Part model, mm, in its own coordinate system. A direction names the side the tool comes from. Round coordinates to 2 decimals unless told otherwise and drop trailing zeros. Loops run counter-clockwise (first coordinate to the right, second up) from the corner with the lowest first, then second, coordinate; pieces in that order, holes last. Notation, with made-up numbers: M 16,-29.5 L 26,-29.5 A16 cw 26,-5.5 Z; hole C -23,-37.75 d7. An arc over 180 degrees is marked long. Write each question's results on one line, items separated by ' | '.
from build123d import *

# Parameters (mm, degrees)
SKETCH1_R           = 1.249999999
BOSS_EXTRUDE1_DEPTH = 6.35


with BuildPart() as part:
    # Sketch1 → Boss-Extrude1 (new body)
    with BuildSketch(Plane.XY):
        with BuildLine():
            Line((200.750613804, 258.978854223), (200.750613804, 219.828854223))
            ThreePointArc((200.750613804, 219.828854223), (201.680549774, 217.583790192), (203.925613804, 216.653854223))
            Line((203.925613804, 216.653854223), (221.575613802, 216.653854223))
            ThreePointArc((221.575613802, 216.653854223), (223.820677833, 217.583790192), (224.750613802, 219.828854223))
            Line((224.750613802, 219.828854223), (224.750613802, 258.978854223))
            ThreePointArc((224.750613802, 258.978854223), (223.820677833, 261.223918253), (221.575613802, 262.153854223))
            Line((221.575613802, 262.153854223), (203.925613804, 262.153854223))
            ThreePointArc((203.925613804, 262.153854223), (201.680549774, 261.223918253), (200.750613804, 258.978854223))
        make_face()
        with Locations((211.950613802, 247.891354224)):
            Circle(SKETCH1_R, mode=Mode.SUBTRACT)
        with Locations((211.950613802, 257.416354224)):
            Circle(SKETCH1_R, mode=Mode.SUBTRACT)
        with BuildLine():
            Line((203.700613802, 221.203854223), (203.700613802, 224.103854225))
            ThreePointArc((203.700613802, 224.103854225), (206.250613802, 226.653854225), (208.800613803, 224.103854225))
            Line((208.800613803, 224.103854225), (208.800613803, 221.203854223))
            ThreePointArc((208.800613803, 221.203854223), (206.250613802, 218.653854223), (203.700613802, 221.203854223))
        make_face(mode=Mode.SUBTRACT)
        with BuildLine():
            Line((216.700613804, 224.103854225), (216.700613804, 221.203854223))
            ThreePointArc((216.700613804, 221.203854223), (219.250613803, 218.653854224), (221.800613802, 221.203854223))
            Line((221.800613802, 221.203854223), (221.800613802, 224.103854225))
            ThreePointArc((221.800613802, 224.103854225), (219.250613803, 226.653854224), (216.700613804, 224.103854225))
        make_face(mode=Mode.SUBTRACT)
    extrude(amount=BOSS_EXTRUDE1_DEPTH)


solid = part.part
Item 1: Band-saw the part on C-C on z = 3. Give the cut face in (x, y) (3 decimals), and give its area (3 significant figures).
Filled sheet:
outline: M 200.751,219.829 A3.175 ccw 203.926,216.654 L 221.576,216.654 A3.175 ccw 224.751,219.829 L 224.751,258.979 A3.175 ccw 221.576,262.154 L 203.926,262.154 A3.175 ccw 200.751,258.979 Z; hole M 203.701,221.204 A2.55 ccw 208.801,221.204 L 208.801,224.104 A2.55 ccw 203.701,224.104 Z; hole C 211.951,247.891 d2.5; hole C 211.951,257.416 d2.5; hole M 216.701,221.204 A2.55 ccw 221.801,221.204 L 221.801,224.104 A2.55 ccw 216.701,224.104 Z | area: 1,000 mm^2
Item 2: Wall check: L1, parallel to Y at x = 212, z = 6.25; L2, parallel to X at y = 223, z = 4.75; L3, parallel to X at y = 226, z = 4. Give the ranges that are in metal, low to high.
Filled sheet:
L1: 216.65 to 246.64, 249.14 to 256.17, 258.67 to 262.15 | L2: 200.75 to 203.7, 208.8 to 216.7, 221.8 to 224.75 | L3: 200.75 to 204.55, 207.96 to 217.55, 220.96 to 224.75
Item 3: Band-saw the part on A-A on y = 223.5. Give the cut face in (x, z).
Filled sheet:
outline: M 200.75,0 L 203.7,0 L 203.7,6.35 L 200.75,6.35 Z; M 208.8,0 L 216.7,0 L 216.7,6.35 L 208.8,6.35 Z; M 221.8,0 L 224.75,0 L 224.75,6.35 L 221.8,6.35 Z
Item 4: Two-plate mould, pull along Y, no slides. Class faces 3 (the cylindrical face through (219.195, 218.654, 3.131)), 4 (the cylindrical face through (201.656, 217.609, 3.131)), 5 (the flat face through (208.801, 223, 3)), 6 (the flat face through (224.751, 239, 3)): +Y half, -Y half, draft (parallel to the pull), parting line (faces both ways), or undercut.
Filled sheet:
face 3: undercut | face 4: -Y half | face 5: undercut | face 6: draft
Item 5: Band-saw the part on B-B on x = 205.5. Give the cut face in (y, z), and give its area (3 significant figures).
Filled sheet:
outline: M 216.65,0 L 218.77,0 L 218.77,6.35 L 216.65,6.35 Z; M 226.54,0 L 262.15,0 L 262.15,6.35 L 226.54,6.35 Z | area: 240 mm^2
Item 6: Which spindle directions (+Z, -Z, +X, -X, +Y, -Y) get a long thin tool onto all of the face, cutting with end or side? Do faces 1 (the flat face through (213, 240, 6.35)), 2 (the flat face through (216.701, 223, 3)). Say none if no direction does.
Filled sheet:
face 1: +Z, +X, -X, +Y, -Y | face 2: +Z, -Z
Item 7: Band-saw the part on D-D on x = 219.5. Give the cut face in (y, z), and give its area (3 significant figures).
Filled sheet:
outline: M 216.65,0 L 218.67,0 L 218.67,6.35 L 216.65,6.35 Z; M 226.64,0 L 262.15,0 L 262.15,6.35 L 226.64,6.35 Z | area: 238 mm^2
